Autodesk Inventor part; units mm, degrees
ref_plane "YZ Plane" through (0, 0, 0) normal (1, 0, 0) x (0, 1, 0)
ref_plane "XZ Plane" through (0, 0, 0) normal (0, 1, 0) x (-1, 0, 0)
ref_plane "XY Plane" through (0, 0, 0) normal (0, 0, 1) x (1, 0, 0)
sketch "Sketch1" plane through (0, 0, 0) normal (0, 1, 0) x (-1, 0, 0)
  circle A0 centre (0, 0) radius 2
  dimension "d0" = 4
extrude "Extrusion1" add sketch "Sketch1" along normal blind 58 and the other way blind 3
sketch "Sketch2" plane through (0, 0, 0) normal (0, 1, 0) x (-1, 0, 0)
  circle A0 centre (0, 0) radius 1.5
  circle A1 centre (0, 0) radius 2
  dimension "d3" = 3
  dimension "d4" = 4
extrude "Extrusion2" cut sketch "Sketch2" along normal blind 6.54 and the other way blind 3
thread "Thread1"
thread "Thread2"
sketch "Sketch3" plane through (0, 58, 0) normal (0, 1, 0) x (1, 0, 0)
  circle A0 centre (0, 0) radius 1.5
  circle A1 centre (0, 0) radius 2
  dimension "d11" = 3
  dimension "d12" = 4
extrude "Extrusion3" cut sketch "Sketch3" against normal blind 5
thread "Thread3"
properties part number "Rod Design"
CAD build for the part. Positions are in the model's coordinates, mm. A direction names the side the tool comes from. Give positions to 0.01 mm unless a question says otherwise; leave off trailing zeros. Order: outer loops, then holes, each group sorted by start corner. A loop starts at its lowest first (then second) coordinate and runs counter-clockwise, first axis right, second up.
(1) Saw through at A-A, the plane z = 0. Give the cut face in (x, y).
(2) Saw through at C-C, the plane y = 18. Give the cut face in (x, z), then the cut area to 3 significant figures.
(3) Drill centre lines: L1, parallel to Y at x = -1.25, z = -1.2; L2, parallel to X at y = 28, z = 0.15; L3, parallel to X at y = 36, z = 1.1. Where is each one in solid material? Low to high.
(4) Tool access for faces 1 (the cylindrical face through (0, 29, 2)), 2 (the cylindrical face through (1.5, 1.7, -0.07)), 3 (the cylindrical face through (-1.5, 55.54, -0.07)): list every direction of +Z, -Z, +X, -X, +Y, -Y with a clear straight run to the whole face (end or side of a thin tool).
(5) Saw through at D-D, the plane y = 4. Give the cut face in (x, z), then the cut area to 3 significant figures.
(6) Saw through at B-B, the plane x = -0.45. Give the cut face in (y, z).
Results found:
1. outline: (-2, 6.54) - (-1.5, 6.54) - (-1.5, -3) - (1.5, -3) - (1.5, 6.54) - (2, 6.54) - (2, 53) - (1.5, 53) - (1.5, 58) - (-1.5, 58) - (-1.5, 53) - (-2, 53) - close
2. outline: circle Ø4 at (0, 0)
2. area: 12.6 mm2
3. L1: y = 6.54 to 53
3. L2: x = -1.99 to 1.99
3. L3: x = -1.67 to 1.67
4. face 1: +Y, -Y
4. face 2: -Y
4. face 3: +Y
5. outline: circle Ø3 at (0, 0)
5. area: 7.07 mm2
6. outline: (-3, -1.43) - (6.54, -1.43) - (6.54, -1.95) - (53, -1.95) - (53, -1.43) - (58, -1.43) - (58, 1.43) - (53, 1.43) - (53, 1.95) - (6.54, 1.95) - (6.54, 1.43) - (-3, 1.43) - close
